The model under review builds one solid part; all positions refer to its coordinate system, in mm. Face numbers are marked on the shaded views. A direction names the side the tool comes from. Coordinates: 2 decimals unless noted, no trailing zeros.
```python
from build123d import *

# Parameters (mm, degrees)
F0_R     = 8.8190251349
F1_DEPTH = 25
F2_COUNT = 12


# Not quite as in the source:
# - a feature names something its author has since deleted; it is built from what else it names


with BuildPart() as f1:
    # F0 (on Front) → F1 (new body)
    with BuildSketch(Plane.XZ):
        with BuildLine():
            ThreePointArc((-5.8511671906, 26.2154592323), (-16.7976364993, -20.9601018196), (26.8605, 0))
            ThreePointArc((26.8605, 0), (20.0037882945, 17.9258169722), (2.9342950433, 26.6997448087))
            ThreePointArc((2.9342950433, 26.6997448087), (-1.4784007951, 26.8197835811), (-5.8511671906, 26.2154592323))
        make_face()
        Circle(F0_R, mode=Mode.SUBTRACT)
        with BuildLine():
            ThreePointArc((-5.8511671906, 26.2154592323), (-1.4784007951, 26.8197835811), (2.9342950433, 26.6997448087))
            ThreePointArc((2.9342950433, 26.6997448087), (2.7429832933, 29.2065995461), (2.0526051191, 31.6240980128))
            ThreePointArc((2.0526051191, 31.6240980128), (0.8166449435, 34.1202908544), (-0.8038354447, 36.3858193952))
            ThreePointArc((-0.8038354447, 36.3858193952), (-2.1425207788, 36.9553506751), (-3.3954147249, 36.215958315))
            ThreePointArc((-3.3954147249, 36.215958315), (-4.7063208649, 33.7582965503), (-5.6058886832, 31.122133809))
            ThreePointArc((-5.6058886832, 31.122133809), (-5.9726089783, 28.6809978257), (-5.8511671906, 26.2154592323))
        make_face()
    extrude(amount=F1_DEPTH)

    # F2: F1 ×12 about axis
    f2_axis = Axis((0, 0, 0), (0, 1, 0))


with BuildPart() as f1_1:
    add(f1.part)
    for i in range(1, F2_COUNT):
        add(f1.part.rotate(f2_axis, i * 360 / F2_COUNT))


solid = f1_1.part
```
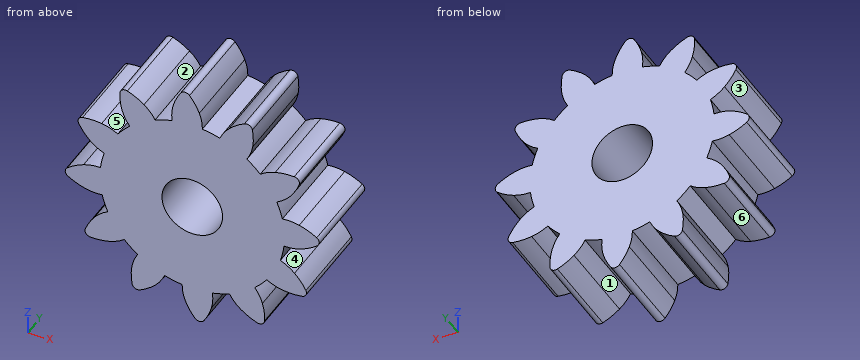
Item 1: To check wall thickness, follow line 1 along Z through (x, y) = (0, -13.5); line 2 along Z through (x, y) = (1.5, -14.5); line 3 along X through (y, z) = (-6, -8). State the ranges of each line that lie inside material, in increasing order.
Solved:
line 1: z = -35.36 to -8.82, 8.82 to 35.36
line 2: z = -36.87 to -8.69, 8.69 to 32.87
line 3: x = -25.64 to -3.71, 3.71 to 25.64
Item 2: Mouldability with a two-part tool opening along Z and no side actions: class the marked faces 4, 5 and 6 as pulls with the +Z half, pulls with the -Z half, needs draft (parallel to the pull), parting line crosses it, or undercut.
Solved:
face 4: undercut
face 5: pulls with the +Z half
face 6: pulls with the -Z half
Item 3: For pin 1 (12 mm diameter, centred on y = -6, z = -16.5, fed in from +X); pin 2 (6 mm diameter, centred on x = 0.5, z = -3, fed in from +Y); pin 3 (1 mm diameter, centred on y = -8, z = 19, fed in from +X); pin 4 (2 mm diameter, centred on x = 27.5, y = -10.5, fed in from +Z), all flat-tipped, find the tip position at first contact; note any pin that passes through.
Solved:
pin 1: stops at x = 33.24
pin 2: passes through
pin 3: stops at x = 31.2
pin 4: stops at z = 21.06
Item 4: Machinability: for the marked faces 1, 2 and 3, which of the approach directions +Z, -Z, +X, -X, +Y, -Y give a long, thin tool a straight path to every point of the face, cutting with its end or side? Answer none if there is none.
Solved:
face 1: -Z, +Y, -Y
face 2: +Z, +Y, -Y
face 3: -X, +Y, -Y
